Model file for the job. Use its own axes, mm. Coordinates: 2 decimals unless noted, no trailing zeros. Loops run counter-clockwise (first coordinate to the right, second up) from the corner with the lowest first, then second, coordinate; pieces in that order, holes last. Notation, with made-up numbers: M 26,-21 L 59,-21 A15 ccw 59,2 Z; hole C 20.5,19.25 d3. An arc over 180 degrees is marked long. Write item = value, one per line. Start each with the question number.
Autodesk Fusion 360 part; units mm, degrees
sketch "Sketch1" plane through (0, 0, 0) normal (0, 1, 0) x (1, 0, 0)
  line L0 (0, 0) -> (0, -50.0731) construction
  line L1 (-71.5, 0) -> (71.5, 0)
  line L2 (71.5, 0) -> (71.5, -40)
  line L3 (71.5, -40) -> (-71.5, -40)
  line L4 (-71.5, -40) -> (-71.5, 0)
  line L5 (-71.5, -20) -> (71.5, -20) construction
  line L6 (-65.5, -34) -> (65.5, -34) construction
  line L7 (65.5, -34) -> (65.5, -6) construction
  line L8 (65.5, -6) -> (-65.5, -6) construction
  line L9 (-65.5, -6) -> (-65.5, -34) construction
  circle A0 centre (-65.5, -34) radius 2
  circle A1 centre (65.5, -34) radius 2
  circle A2 centre (65.5, -6) radius 2
  circle A3 centre (-65.5, -6) radius 2
  circle A4 centre (37.5, -20) radius 9
  circle A5 centre (-37.5, -20) radius 9
  circle A6 centre (0, -20) radius 9
  dimension "d1" = 143
  dimension "d2" = 40
  dimension "d3" = 71.5
  dimension "d4" = 40
  dimension "d5" = 6
  dimension "d6" = 6
  dimension "d7" = 6
  dimension "d8" = 6
  dimension "d9" = 4
  dimension "d10" = 4
  dimension "d11" = 4
  dimension "d12" = 4
  dimension "d16" = 18
  dimension "d17" = 18
  dimension "d25" = 18
  dimension "d26" = 37.5
  dimension "d27" = 37.5
extrude "Extrude1" add sketch "Sketch1" along normal blind 2
equation "d3 = d1 / 2"
equation "d4 = d2"
equation "d6 = d5"
equation "d8 = d7"
equation "d10 = d9"
equation "d11 = d9"
equation "d12 = d9"
equation "HoleSpread = 75 mm"
equation "HoleDia = 18 mm"
equation "d16 = HoleDia"
equation "d17 = HoleDia"
equation "d25 = HoleDia"
equation "d26 = HoleSpread / 2"
equation "d27 = HoleSpread / 2"
Item 1: Cut at B-B (x = -37.5). Give the cut face in (y, z).
Item 2: Probe L1, parallel to Z at x = -65.5, y = 0.8; L2, parallel to X at y = 1.05, z = 6; L3, parallel to X at y = 0.4, z = 20. List the from-to ranges inside material, lowest first.
Item 3: Cut at D-D (y = 1.35). Give the cut face in (x, z), plus the area to 3 significant figures.
Item 4: Cut at A-A (x = 65.5). Give the cut face in (y, z), plus the area to 3 significant figures.
Item 5: Pull direction X, two halves, no side cores. Call faces 1 (the flat face through (-1, 0, 10.8)), 2 (the cylindrical face through (28.51, 0.99, 20.4)), 3 (the cylindrical face through (-1.172, 0.986, 28.923)): +X half, -X half, draft (parallel to the pull), parting line (faces both ways), or undercut.
Item 6: Cut at C-C (z = 34). Give the cut face in (x, y), plus the area to 3 significant figures.
Reported:
q1.outline = M 0,0 L 2,0 L 2,11 L 0,11 Z; M 0,29 L 2,29 L 2,40 L 0,40 Z
q2.L1 = 0 to 4, 8 to 32, 36 to 40
q2.L2 = -71.5 to -67.5, -63.5 to 63.5, 67.5 to 71.5
q2.L3 = -71.5 to -46.5, -28.5 to -9, 9 to 28.5, 46.5 to 71.5
q3.outline = M -71.5,0 L 71.5,0 L 71.5,40 L -71.5,40 Z; hole C -65.5,6 d4; hole C -65.5,34 d4; hole C -37.5,20 d18; hole C 0,20 d18; hole C 37.5,20 d18; hole C 65.5,6 d4; hole C 65.5,34 d4
q3.area = 4,910 mm^2
q4.outline = M 0,0 L 2,0 L 2,4 L 0,4 Z; M 0,8 L 2,8 L 2,32 L 0,32 Z; M 0,36 L 2,36 L 2,40 L 0,40 Z
q4.area = 64.0 mm^2
q5.face_1 = draft
q5.face_2 = undercut
q5.face_3 = undercut
q6.outline = M -71.5,0 L -67.5,0 L -67.5,2 L -71.5,2 Z; M -63.5,0 L 63.5,0 L 63.5,2 L -63.5,2 Z; M 67.5,0 L 71.5,0 L 71.5,2 L 67.5,2 Z
q6.area = 270 mm^2
